```python
from build123d import *

# Parameters (mm, degrees)
ESKIZ_KONTUR_W        = 5.2
ESKIZ_KONTUR_H        = 9.2
PLASTINA_DEPTH        = 5
OTVERSTIYA_DEPTH      = 85.528105852
OTVERSTIYA_DEPTH_BACK = 85.528105852
ESKIZ_OTVERSTIYA_R    = 1.65
ESKIZ_OTVERSTIYA_R_2  = 2.15


with BuildPart() as part:
    # Eskiz_kontur → Plastina (new body)
    with BuildSketch(Plane.XY):
        with BuildLine():
            Line((21.958964111, 51.343070401), (24.999994111, 4.01e-07))
            Line((24.999994111, 4.01e-07), (17, 4.01e-07))
            Line((17, 4.01e-07), (17, -5))
            Line((17, -5), (5, -5))
            Line((5, -5), (5, 0))
            Line((5, 0), (-7.35, 0))
            Line((-7.35, 0), (-7.35, 4.5))
            Line((-7.35, 4.5), (-6.1, 4.5))
            Line((-6.1, 4.5), (-6.1, 7.1))
            Line((-6.1, 7.1), (-7.35, 7.1))
            Line((-7.35, 7.1), (-7.35, 10))
            Line((-7.35, 10), (-10.65, 10))
            Line((-10.65, 10), (-10.65, 7.1))
            Line((-10.65, 7.1), (-11.9, 7.1))
            Line((-11.9, 7.1), (-11.9, 4.5))
            Line((-11.9, 4.5), (-10.65, 4.5))
            Line((-10.65, 4.5), (-10.65, 0))
            Line((-10.65, 0), (-23, 0))
            Line((-23, 0), (-23, -5))
            Line((-23, -5), (-35, -5))
            Line((-35, -5), (-35, 0))
            Line((-35, 0), (-42, 0))
            Line((-42, 0), (-43.99513, 57.7208))
            ThreePointArc((-43.99513, 57.7208), (-42.217170806, 63.034563621), (-37.389183787, 65.878463067))
            Line((-37.389183787, 65.878463067), (-3.820263787, 71.665773067))
            ThreePointArc((-3.820263787, 71.665773067), (13.620063981, 67.276975245), (21.958964111, 51.343070401))
        make_face()
        with Locations((-35.5, 16.5)):
            Rectangle(ESKIZ_KONTUR_W, ESKIZ_KONTUR_H, mode=Mode.SUBTRACT)
        with BuildLine():
            Line((10, 34), (-20, 34))
            ThreePointArc((-20, 34), (-26, 28), (-20, 22))
            Line((-20, 22), (10, 22))
            ThreePointArc((10, 22), (16, 28), (10, 34))
        make_face(mode=Mode.SUBTRACT)
    extrude(amount=PLASTINA_DEPTH)

    # Eskiz_otverstiya → Otverstiya (cut, two sides: drawn at the far end of the back side and taken through both)
    with BuildSketch(Plane.XY.offset(-OTVERSTIYA_DEPTH_BACK)):
        with Locations((-35.5, 7.5)):
            Circle(ESKIZ_OTVERSTIYA_R)
        with Locations((0, 50)):
            Circle(ESKIZ_OTVERSTIYA_R_2)
    extrude(amount=OTVERSTIYA_DEPTH + OTVERSTIYA_DEPTH_BACK, mode=Mode.SUBTRACT)


solid = part.part
```
The model under review builds one solid part; all positions refer to its coordinate system, in mm. A direction names the side the tool comes from. Give positions to 0.01 mm unless a question says otherwise; leave off trailing zeros. Write each loop counter-clockwise with the first axis right and the second up, starting at its lowest first coordinate (ties: lowest second). Pieces come first, ordered by that corner, then holes.
(1) Consider section B-B, the plane y = 20. Give the boundary of the cut face in (x, z).
(2) To check wall thickness, follow L1, parallel to Y at x = 0, z = 3.75; L2, parallel to Y at x = -35.5, z = 2.45; L3, parallel to X at y = -0.5, z = 4.6. State the ranges of each line that lie inside material, in increasing order.
(3) Consider section A-A, the plane x = 0. Give the boundary of the cut face in (y, z), and give its area (4 significant figures).
(4) Tool access review of faces 1 (the flat face through (21, 0, 2)), 2 (the cylindrical face through (16, 28, 2)), 3 (the flat face through (-35, -3, 2)), 4 (the flat face through (-9, 10, 2)): name each direction out of +Z, -Z, +X, -X, +Y, -Y from which nothing blocks a thin tool from reaching the whole face with its end or side.
(5) Consider section C-C, the plane z = 2.7. Give the number of separate pieces and of enclosed holes in the cut face, and give its area (3 significant figures).
(6) Consider section D-D, the plane y = 28. Give the boundary of the cut face in (x, z).
(7) The part is to be moulded in two halves that separate along Y. For faces 5 (the flat face through (-29, -5, 2)), 6 (the cylindrical face through (-37.15, 7.57, 2.47)), 7 (the flat face through (-5, 34, 2)), 8 (the flat face through (-7.35, 2, 2)), say which applies: released by +Y, released by -Y, zero draft, split by the parting line, or undercut.
(8) For P1, Ø2, axis at y = 62.5, z = 1, coming from the +X side (3 decimals); P2, Ø3, axis at y = 9, z = 3, coming from the -X side; P3, Ø3, axis at y = 6, z = 1.5, coming from the -X side, all flat-tipped, find the tip position at first contact; note any pin that passes through.
Returned:
1. outline: (-42.69, 0) - (-38.1, 0) - (-38.1, 5) - (-42.69, 5) - close; (-32.9, 0) - (23.82, 0) - (23.82, 5) - (-32.9, 5) - close
2. L1: y = 0 to 22, 34 to 47.85, 52.15 to 72
2. L2: y = 0 to 5.85, 9.15 to 11.9, 21.1 to 66.2
2. L3: x = -35 to -23, 5 to 17
3. outline: (0, 0) - (22, 0) - (22, 5) - (0, 5) - close; (34, 0) - (47.85, 0) - (47.85, 5) - (34, 5) - close; (52.15, 0) - (72, 0) - (72, 5) - (52.15, 5) - close
3. area: 278.5 mm2
4. face 1: +Z, -Z, +X, -Y
4. face 2: +Z, -Z
4. face 3: +Z, -Z, -X, -Y
4. face 4: +Z, -Z, -Y
5. separate pieces: 1
5. enclosed holes: 4
5. area: 4,040 mm2
6. outline: (-42.97, 0) - (-26, 0) - (-26, 5) - (-42.97, 5) - close; (16, 0) - (23.34, 0) - (23.34, 5) - (16, 5) - close
7. face 5: released by -Y
7. face 6: undercut
7. face 7: undercut
7. face 8: zero draft
8. P1: stops at x = 18.755
8. P2: stops at x = -42.36
8. P3: stops at x = -42.26
